from build123d import *

# Parameters (mm, degrees)
F2_W     = 39
F2_H     = 39
F3_DEPTH = 20
F5_R     = 7
F6_R     = 1.6
F7_DEPTH = 20.001
F7_TAPER = -5


with BuildPart() as f1:
    # F0 (on Top) → F1 (revolve)
    with BuildSketch(Plane.XY):
        with BuildLine():
            Line((0, 0), (36, 0))
            ThreePointArc((36, 0), (18, 18), (0, 0))
        make_face()
    revolve(axis=Axis((18, 0, 0), (1, 0, 0)))


with BuildPart() as f3:
    # F2 (on Top) → F3 (new body)
    with BuildSketch(Plane.XY):
        with Locations((18, 0)):
            Rectangle(F2_W, F2_H)
    extrude(amount=-F3_DEPTH)

    # F4: cut F1
    add(f1.part, mode=Mode.SUBTRACT)

    # F5
    f5_edges = [f3.edges().sort_by_distance(p)[0] for p in [
        (-1.5, -19.5, -10),
        (37.5, -19.5, -10),
        (37.5, 19.5, -10),
        (-1.5, 19.5, -10),
    ]]
    fillet(f5_edges, radius=F5_R)

    # F6 (on face) → F7 (cut, through all)
    with BuildSketch(Plane.XY):
        with Locations((32.5663996924, 14.5663996924)):
            Circle(F6_R)
        with Locations((3.4336003076, 14.5663996924)):
            Circle(F6_R)
        with Locations((3.4336003076, -14.5663996924)):
            Circle(F6_R)
        with Locations((32.5663996924, -14.5663996924)):
            Circle(F6_R)
    extrude(amount=-F7_DEPTH, taper=F7_TAPER, mode=Mode.SUBTRACT)


solid = f3.part
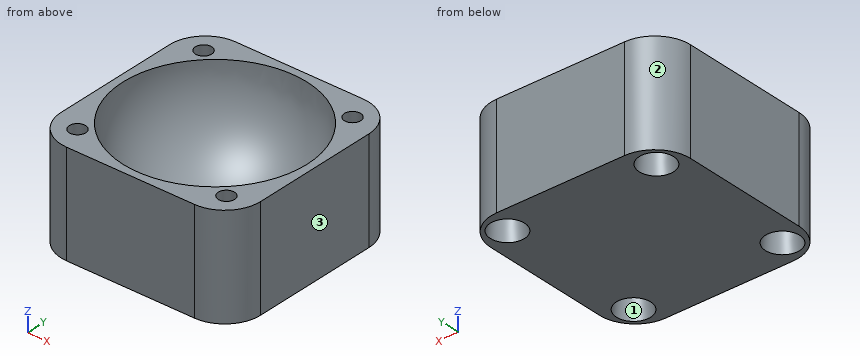
The listing builds one solid part. Answer for the finished solid, in the listing's coordinates (mm). Face numbers are marked on the shaded views. Give positions to 0.01 mm unless a question says otherwise; leave off trailing zeros. Loops run counter-clockwise (first coordinate to the right, second up) from the corner with the lowest first, then second, coordinate; pieces in that order, holes last. Notation, with made-up numbers: (64.25, 10) - (101.25, 10) arc R27 cw to (101.25, 26) - close; hole circle Ø9 at (-39, 28.5). An arc over 180 degrees is marked (long way). Use one line per item in the form item = value.
1. Find the intervals of material crossed by line 1 along Y through (x, z) = (30.5, -18); line 2 along X through (y, z) = (-16, -4.75); line 3 along X through (y, z) = (12, -14.75), in increasing order. Write a range as [from, to].
Calculated:
line_1 = [-19.5, -16.98], [-12.16, 12.16], [16.98, 19.5]
line_2 = [-0.56, 2.02], [4.85, 11.26], [24.74, 31.15], [33.98, 36.56]
line_3 = [-1.5, 2.1], [4.76, 31.24], [33.9, 37.5]
2. Section A-A on z = -15.75 is taken. Give the vertices of the cut face in (x, y).
Calculated:
outline = (-1.5, -12.5) arc R7 ccw to (5.5, -19.5) - (30.5, -19.5) arc R7 ccw to (37.5, -12.5) - (37.5, 12.5) arc R7 ccw to (30.5, 19.5) - (5.5, 19.5) arc R7 ccw to (-1.5, 12.5) - close; hole circle Ø5.96 at (3.43, -14.57); hole circle Ø5.96 at (3.43, 14.57); hole circle Ø17.43 at (18, 0); hole circle Ø5.96 at (32.57, -14.57); hole circle Ø5.96 at (32.57, 14.57)
3. Given pin 1 Ø3 at (x, y) = (13.5, -2) entering from +Z, flat-ended and moving along its own axis, determine where the tip first touches the part or whether it passes through.
Calculated:
pin_1 = -16.81
4. Section B-B on x = 18 is taken. Give the vertices of the cut face in (y, z).
Calculated:
outline = (-19.5, -20) - (19.5, -20) - (19.5, 0) - (18, 0) arc R18 cw to (-18, 0) - (-19.5, 0) - close
5. Section D-D on z = -5.75 is taken. Give the vertices of the cut face in (x, y), then the cut area to 3 significant figures.
Calculated:
outline = (-1.5, -12.5) arc R7 ccw to (5.5, -19.5) - (30.5, -19.5) arc R7 ccw to (37.5, -12.5) - (37.5, 12.5) arc R7 ccw to (30.5, 19.5) - (5.5, 19.5) arc R7 ccw to (-1.5, 12.5) - close; hole circle Ø34.11 at (18, 0); hole circle Ø4.21 at (3.43, -14.57); hole circle Ø4.21 at (3.43, 14.57); hole circle Ø4.21 at (32.57, -14.57); hole circle Ø4.21 at (32.57, 14.57)
area = 509 mm^2
6. Section C-C on y = -2 is taken. Give the vertices of the cut face in (x, z).
Calculated:
outline = (-1.5, -20) - (37.5, -20) - (37.5, 0) - (35.89, 0) arc R17.89 cw to (0.11, 0) - (-1.5, 0) - close
7. The mould has two halves that part along Y. Classify the marked faces 1, 2 and 3: pulls with the +Y half, pulls with the -Y half, needs draft (parallel to the pull), parting line crosses it, or undercut.
Calculated:
face_1 = undercut
face_2 = pulls with the +Y half
face_3 = needs draft
